Source: CAD feature listing. Evaluate the final solid. Frame: model axes, mm. A direction names the side the tool comes from. Round coordinates to 2 decimals unless told otherwise and drop trailing zeros. Write each loop counter-clockwise with the first axis right and the second up, starting at its lowest first coordinate (ties: lowest second). Pieces come first, ordered by that corner, then holes. Notation, with made-up numbers: (81, 82) -> (140, 82) arc R23 cw to (140, 116) -> close; hole circle Ø4 at (30, 2.25). An arc over 180 degrees is marked (long way). Return JSON: item names as keys, results as strings. Group by question number.
Autodesk Inventor part; units mm, degrees
ref_plane "YZ Plane" through (0, 0, 0) normal (1, 0, 0) x (0, 1, 0)
ref_plane "XZ Plane" through (0, 0, 0) normal (0, 1, 0) x (-1, 0, 0)
ref_plane "XY Plane" through (0, 0, 0) normal (0, 0, 1) x (1, 0, 0)
sketch "Sketch1" plane through (0, 0, 0) normal (0, 1, 0) x (-1, 0, 0)
  line L0 (0, 0) -> (-304.8, 0)
  line L1 (-304.8, 0) -> (-304.8, -76.2)
  line L2 (-304.8, -76.2) -> (0, -76.2)
  line L3 (0, -76.2) -> (0, 0)
  circle A0 centre (-6.35, -69.85) radius 1.3891
  circle A1 centre (-6.35, -6.35) radius 1.3891
  circle A2 centre (-298.45, -6.35) radius 1.3891
  circle A3 centre (-298.45, -69.85) radius 1.3891
  line L4 (-152.4, -76.2) -> (-152.4, 0)
  line L5 (-304.8, -38.1) -> (0, -38.1)
  line L6 (-127, -50.8) -> (-177.8, -50.8)
  line L7 (-177.8, -50.8) -> (-177.8, -25.4)
  line L8 (-177.8, -25.4) -> (-127, -25.4)
  line L9 (-127, -25.4) -> (-127, -50.8)
  line L10 (-127, -50.8) -> (-177.8, -25.4) construction
  line L11 (-177.8, -50.8) -> (-127, -25.4) construction
  line L12 (-120.65, -57.15) -> (-184.15, -57.15) construction
  line L13 (-184.15, -57.15) -> (-184.15, -19.05) construction
  line L14 (-184.15, -19.05) -> (-120.65, -19.05) construction
  line L15 (-120.65, -19.05) -> (-120.65, -57.15) construction
  circle A4 centre (-120.65, -57.15) radius 1.5875
  circle A5 centre (-184.15, -57.15) radius 1.5875
  circle A6 centre (-120.65, -19.05) radius 1.5875
  circle A7 centre (-184.15, -19.05) radius 1.5875
  point P0 (-152.4, -38.1)
  dimension "d0" = 76.2
  dimension "d1" = 304.8
  dimension "d4" = 2.7781
  dimension "d5" = 6.35
  dimension "d6" = 6.35
  dimension "d7" = 6.35
  dimension "d8" = 6.35
  dimension "d16" = 50.8
  dimension "d17" = 25.4
  dimension "d19" = 6.35
  dimension "d20" = 3.175
extrude "Extrusion1" add sketch "Sketch1" against normal blind 12.7 contours L3 L5 L9 L8 L4 L0 | L4 L8 L7 L5 L1 L0 | L3 L2 L4 L6 L9 L5 | L5 L7 L6 L4 L2 L1 | A0 | A1 | A2 | A3 | A4 | A5 | A6 | A7
hole "Hole1" at (6.35, 0, -69.85) at (298.45, 0, -69.85) at (298.45, 0, -6.35) at (6.35, 0, -6.35) direction (0, -1, 0) diameter 3.2766 end through all countersink diameter 5.715 countersink angle 82
hole "Hole2" at (120.65, 0, -57.15) at (184.15, 0, -57.15) at (184.15, 0, -19.05) at (120.65, 0, -19.05) direction (0, -1, 0) diameter 3.81 end through all
fillet "Fillet1" radius 6.35 4 edges at (127, -6.35, -50.8) (127, -6.35, -25.4) (177.8, -6.35, -25.4) (177.8, -6.35, -50.8)
equation "\"d7\" = d5"
equation "\"d8\" = d6"
properties material "MDF Medium Density Fiberboard"
Item 1: First-contact query: pin 1 Ø4.5 at (x, z) = (298.45, -6.35) entering from +Y; pin 2 Ø5 at (x, z) = (6.35, -69.85) entering from +Y. Flat tips, straight axial feed; report the tip coordinate or a pass-through.
Item 2: Pull-direction query (Z, two-part tool) for faces 3 (the flat face through (155, -6, -76.2)), 4 (the flat face through (0, -6, -39)), 5 (the cylindrical face through (175.99, -6.44, -27.31)); classes: +Z half, -Z half, draft (parallel to the pull), parting line (faces both ways), or undercut.
Item 3: Set-up query: faces 1 (the cylindrical face through (175.89, -6.44, -48.99)), 2 (the flat face through (304.8, -6, -38)). Return all of +Z, -Z, +X, -X, +Y, -Y with unobstructed straight access to the full face (end or side cutting, diameter ignored); none if empty.
Item 4: Cut plane A-A on z = -41.5. Output: boundary loops of the cut face in (x, y), and give its area (3 significant figures).
Item 5: Cut plane B-B on x = 162. Output: boundary loops of the cut face in (y, z), and give its area (3 significant figures).
Item 6: Cut plane C-C on y = -4. Give the number of separate pieces and of enclosed holes in the cut face, and give its area (3 significant figures).
Item 7: Material intervals for probe 1 along Z at (x, y) = (298.45, -4.25); probe 2 along X at (y, z) = (-2.75, -19.05) (3 decimals); probe 3 along X at (y, z) = (-5.5, -70), sorted ascending.
Here are the results:
{
 "1": {"pin 1": "stops at y = -0.7", "pin 2": "stops at y = -0.41"},
 "2": {"face 3": "-Z half", "face 4": "draft", "face 5": "undercut"},
 "3": {"face 1": "+Y, -Y", "face 2": "+Z, -Z, +X, +Y, -Y"},
 "4": {"outline": "(0, -12.7) -> (127, -12.7) -> (127, 0) -> (0, 0) -> close; (177.8, -12.7) -> (304.8, -12.7) -> (304.8, 0) -> (177.8, 0) -> close", "area": "3,230 mm^2"},
 "5": {"outline": "(-12.7, -76.2) -> (0, -76.2) -> (0, -50.8) -> (-12.7, -50.8) -> close; (-12.7, -25.4) -> (0, -25.4) -> (0, 0) -> (-12.7, 0) -> close", "area": "645 mm^2"},
 "6": {"separate pieces": "1", "enclosed holes": "9", "area": "21,900 mm^2"},
 "7": {"probe 1": "z = -76.2 to -71.49, -68.21 to -7.99, -4.71 to 0", "probe 2": "x = 0 to 118.745, 122.555 to 182.245, 186.055 to 304.8", "probe 3": "x = 0 to 4.72, 7.98 to 296.82, 300.08 to 304.8"}
}
